Part print with two shaded views. Sizes in mm from the minimum x, y, z corner. A direction names the side the tool comes from. Round coordinates to 2 decimals unless told otherwise and drop trailing zeros. Write each loop counter-clockwise with the first axis right and the second up, starting at its lowest first coordinate (ties: lowest second). Pieces come first, ordered by that corner, then holes. Notation, with made-up numbers: (82.5, 3.25) - (129.5, 3.25) arc R5 cw to (129.5, 11.25) - close; hole circle Ø5 at (-8, 28.5). An arc over 180 degrees is marked (long way). Answer as a JSON object with one key per item and string values. Group by question number.
Item 1: Which spindle directions (+Z, -Z, +X, -X, +Y, -Y) get a long thin tool onto all of the face, cutting with end or side? Do the marked faces 5 and 6. Say none if no direction does.
Item 2: Probe line 1 (X direction, y = 19, z = 32); line 2 (Y direction, x = 19, z = 19). List the from-to ranges inside material, lowest first. Write a range as from..to.
Item 3: Slice it at C-C, the plane z = 18. List the corners of the cut face in (x, y).
Item 4: Slice it at D-D, the plane x = 33.5. List the corners of the cut face in (y, z), then the cut area to 3 significant figures.
Item 5: Two-plate mould, pull along X, no slides. Class the marked faces 1, 2, 3 and 4: +X half, -X half, draft (parallel to the pull), parting line (faces both ways), or undercut.
Item 6: Flat gauge pins, fed straight in: pin 1 (10 mm diameter, centred on x = 19.5, y = 4.5, fed in from +Z); pin 2 (2 mm diameter, centred on x = 24.5, z = 31.5, fed in from -Y). Where does each tip first touch, or does it go through?
Item 7: Slice it at A-A, the plane y = 19.05. List the corners of the cut face in (x, z), then the cut area to 3 significant figures.
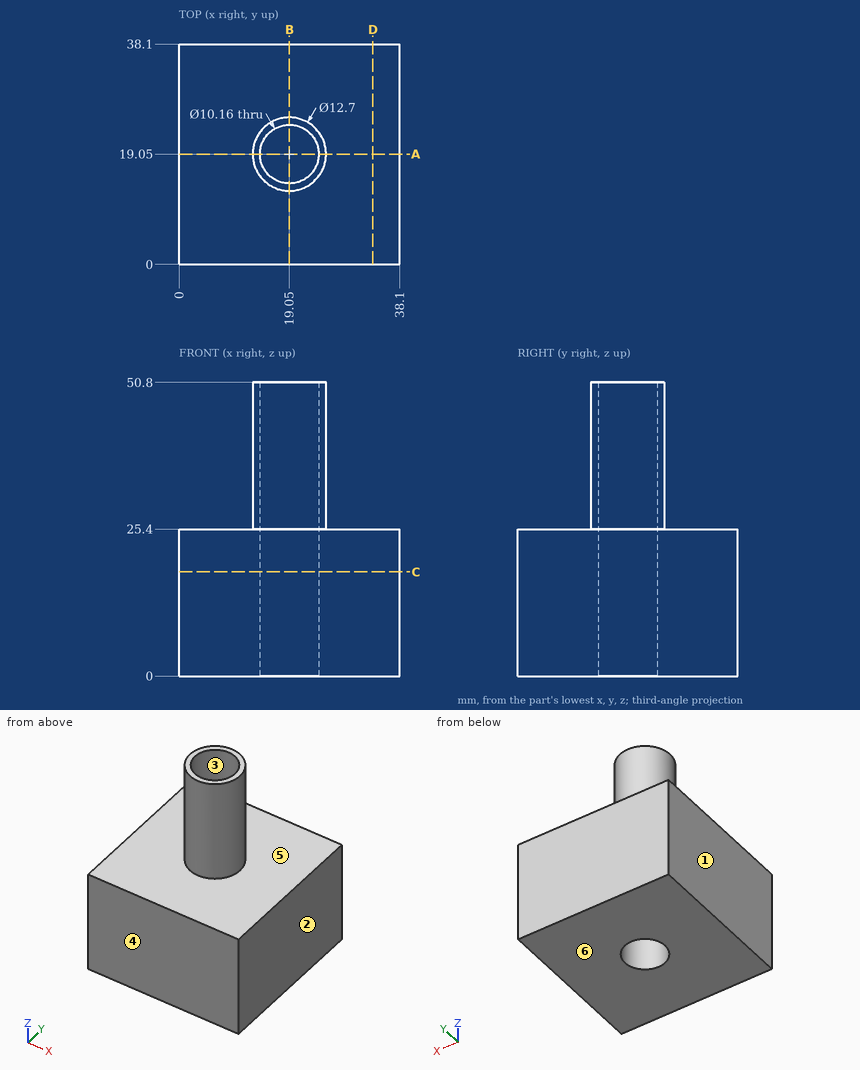
Geometry says:
{
 "1": {"face 5": "+Z", "face 6": "-Z, +X, -X, +Y, -Y"},
 "2": {"line 1": "x = 12.7..13.97, 24.13..25.4", "line 2": "y = 0..13.97, 24.13..38.1"},
 "3": {"outline": "(0, 0) - (38.1, 0) - (38.1, 38.1) - (0, 38.1) - close; hole circle Ø10.16 at (19.05, 19.05)"},
 "4": {"outline": "(0, 0) - (38.1, 0) - (38.1, 25.4) - (0, 25.4) - close", "area": "968 mm^2"},
 "5": {"face 1": "-X half", "face 2": "+X half", "face 3": "undercut", "face 4": "draft"},
 "6": {"pin 1": "stops at z = 25.4", "pin 2": "stops at y = 14.52"},
 "7": {"outline": "(0, 0) - (13.97, 0) - (13.97, 50.8) - (12.7, 50.8) - (12.7, 25.4) - (0, 25.4) - close; (24.13, 0) - (38.1, 0) - (38.1, 25.4) - (25.4, 25.4) - (25.4, 50.8) - (24.13, 50.8) - close", "area": "774 mm^2"}
}
